Could you check a few things on this drawing? It's one solid part, dimensions in mm from its lowest x, y, z. Round coordinates to 2 decimals unless told otherwise and drop trailing zeros. Order: outer loops, then holes, each group sorted by start corner. A loop starts at its lowest first (then second) coordinate and runs counter-clockwise, first axis right, second up. Notation, with made-up numbers: (75, 13) - (79, 13) arc R31 ccw to (79, 46) - close; hole circle Ø9 at (12.5, -5.75). An arc over 180 degrees is marked (long way). Use one line per item in the form item = value.
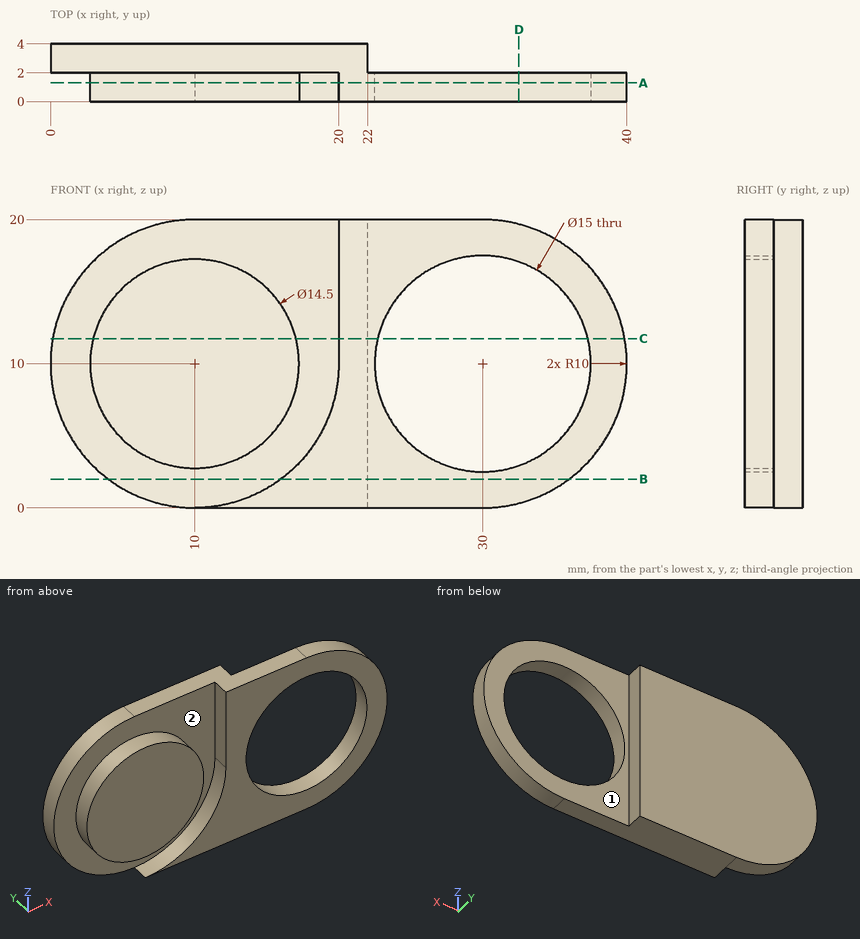
Item 1: Will these pins go through, and if not, where does the flat tip stop? P1, Ø2, axis at x = 24.5, y = 3.5, coming from the -Z side; P2, Ø2, axis at y = 0.5, z = 13, coming from the -X side.
Found:
P1 = through
P2 = 3.03
Item 2: I need wall thicknesses on L1, parallel to Z at x = 30, y = 1.45; L2, parallel to X at y = 1.85, z = 7.5; L3, parallel to Y at x = 27.5, z = 2.5. Which ranges of each line are inside material? Lowest first, please.
Found:
L1 = 0 to 2.5, 17.5 to 20
L2 = 3.19 to 16.81, 19.68 to 22.93, 37.07 to 39.68
L3 = 0 to 2
Item 3: If we mould it in two halves opening along X, with no side actions, what happens to the marked faces 1 and 2? For each: released by +X, released by -X, zero draft, split by the parting line, or undercut.
Found:
face_1 = zero draft
face_2 = undercut
Item 4: Imagine slicing it at B-B on z = 2. Please give me the cut outline in (x, y).
Found:
outline = (4, 2) - (16, 2) - (16, 0) - (36, 0) - (36, 2) - (22, 2) - (22, 4) - (4, 4) - close
Item 5: Imagine slicing it at A-A on y = 1.3. Please give me the cut outline in (x, z), plus the area to 3 significant figures.
Found:
outline = circle Ø14.5 at (10, 10); (10, 0) - (30, 0) arc R10 ccw to (30, 20) - (20, 20) - (20, 10) arc R10 cw to start; hole circle Ø15 at (30, 10)
area = 367 mm2
Item 6: Imagine slicing it at C-C on z = 11.75. Please give me the cut outline in (x, y), plus the area to 3 significant figures.
Found:
outline = (0.15, 2) - (2.96, 2) - (2.96, 0) - (17.04, 0) - (17.04, 2) - (20, 2) - (20, 0) - (22.71, 0) - (22.71, 2) - (22, 2) - (22, 4) - (0.15, 4) - close; (37.29, 0) - (39.85, 0) - (39.85, 2) - (37.29, 2) - close
area = 82.4 mm2
Item 7: Imagine slicing it at D-D on x = 32.5. Please give me the cut outline in (y, z), plus the area to 3 significant figures.
Found:
outline = (0, 0.32) - (2, 0.32) - (2, 2.93) - (0, 2.93) - close; (0, 17.07) - (2, 17.07) - (2, 19.68) - (0, 19.68) - close
area = 10.4 mm2
